The figure shows three views and two pictorial views of one solid part (mm, origin at its lowest corner). Answer the questions. A direction names the side the tool comes from. Round coordinates to 2 decimals unless told otherwise and drop trailing zeros. Order: outer loops, then holes, each group sorted by start corner. A loop starts at its lowest first (then second) coordinate and runs counter-clockwise, first axis right, second up. Notation, with made-up numbers: (-35.75, 33.5) - (9.25, 33.5) arc R21 ccw to (9.25, 65.5) - close; hole circle Ø6 at (24, -36.75). An arc over 180 degrees is marked (long way). Answer as a JSON object with one key per item and string values. Group by question number.
Q1. Consider line 1 (Z direction, x = 0.75, y = 6.75); line 2 (Y direction, x = 6.75, z = 11.5); line 3 (Y direction, x = 6.5, z = 10.75). Determine where each line is inside the solid, lowest interval first.
Q2. A cutting plane is placed at C-C on z = 6. Determine the outline of the cut face in (x, y).
Q3. A tool of negligible diameter and unlimited length cuts with its end or side. For the marked faces 1 and 2, from which of +Z, -Z, +X, -X, +Y, -Y can it reach the whole face along a straight path? Write none if from no direction.
Q4. A cutting plane is placed at A-A on y = 5. Determine the outline of the cut face in (x, z), and give its area (3 significant figures).
Q5. Given pin 1 Ø1 at (y, z) = (7, 11.5) entering from +X; pin 2 Ø4 at (y, z) = (4, 10.5) entering from -X; pin 3 Ø5 at (y, z) = (3.5, 18) entering from +X; pin 4 Ø1.5 at (x, z) = (8, 5) entering from +Y, each flat-ended and moving along its own axis, determine where each tip first touches the part or whether it passes through.
Q6. A cutting plane is placed at D-D on z = 17. Determine the outline of the cut face in (x, y), and give its area (3 significant figures).
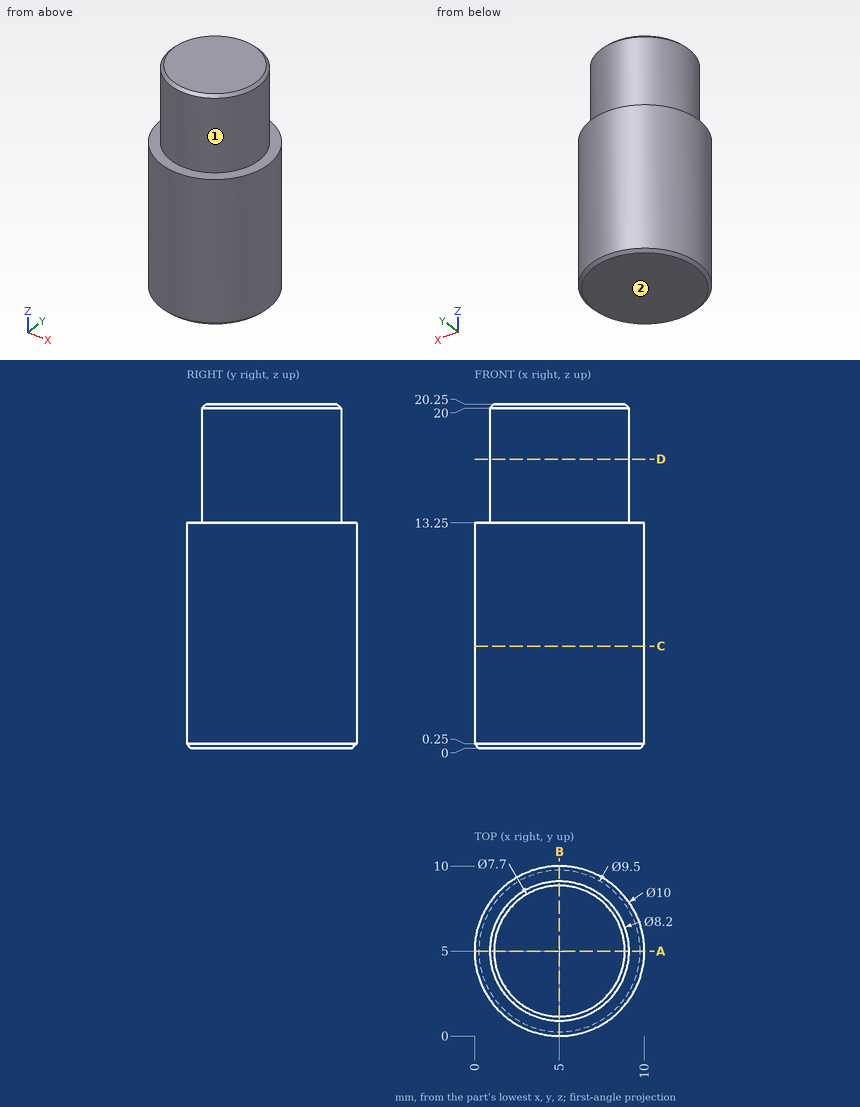
Result set:
{
 "1": {"line 1": "z = 0 to 13.25", "line 2": "y = 0.32 to 9.68", "line 3": "y = 0.23 to 9.77"},
 "2": {"outline": "circle Ø10 at (5, 5)"},
 "3": {"face 1": "+Z", "face 2": "-Z, +X, -X, +Y, -Y"},
 "4": {"outline": "(0, 0.25) - (0.25, 0) - (9.75, 0) - (10, 0.25) - (10, 13.25) - (9.1, 13.25) - (9.1, 20) - (8.85, 20.25) - (1.15, 20.25) - (0.9, 20) - (0.9, 13.25) - (0, 13.25) - close", "area": "190 mm²"},
 "5": {"pin 1": "stops at x = 9.77", "pin 2": "stops at x = 0", "pin 3": "stops at x = 9.1", "pin 4": "stops at y = 9.47"},
 "6": {"outline": "circle Ø8.2 at (5, 5)", "area": "52.8 mm²"}
}
